```python
from build123d import *

# Parameters (mm, degrees)
SKETCH2_R = 2.5


with BuildPart() as part:
    # Sweep1: sweep along a path in Sketch1
    with BuildLine(Plane(origin=(0, 0, 0), x_dir=(1, 0, 0), z_dir=(0, 1, 0))) as sweep1_path:
        Line((0, 0), (0, 65))
        ThreePointArc((0, 65), (4.393398282, 75.606601718), (15, 80))
        Line((15, 80), (215, 80))
        ThreePointArc((215, 80), (225, 70), (215, 60))
        Line((215, 60), (185, 60))
        ThreePointArc((185, 60), (172.034701688, 62.946330384), (161.616073533, 71.206597355))
    # Sketch2 → Sweep1 (sweep)
    with BuildSketch(Plane.XY):
        Circle(SKETCH2_R)
    sweep(path=sweep1_path.line)


solid = part.part
```
Read the model definition and answer for the solid it produces. Units are mm, in the model's axes. A direction names the side the tool comes from. Round coordinates to 2 decimals unless told otherwise and drop trailing zeros. Write each loop counter-clockwise with the first axis right and the second up, starting at its lowest first coordinate (ties: lowest second). Pieces come first, ordered by that corner, then holes. Notation, with made-up numbers: (35, 74) -> (86, 74) arc R17 ccw to (86, 101) -> close; hole circle Ø8 at (55, 35.25). An arc over 180 degrees is marked (long way). Answer in a Markdown table with one row per item. Add a question column.
1) Given P1, Ø1.5, axis at x = 93, y = -1, coming from the -Z side, flat-ended and moving along its own axis, determine where the tip first touches the part or whether it passes through.
2) Which of the six approach directions +Z, -Z, +X, -X, +Y, -Y give full straight-line access (tool end or side, diameter ignored) to faces 1 (the face through (161.589, 0.035, -71.185)), 2 (the face through (116.4, -0.1, -82.5))?
3) Find section B-B, the plane z = -21.5. Determine the outline of the cut face in (x, y).
4) Find section A-A, the plane y = 0. Determine the outline of the cut face in (x, z).
5) Determine the mould class of faces 3 (the face through (0, 0, 0)), 4 (the face through (-0.54, 2.44, -32.96)), 5 (the face through (199.79, 0.96, -62.31)) for opening direction Z: pulls with the +Z half, pulls with the -Z half, needs draft (parallel to the pull), parting line crosses it, or undercut.
6) Find section C-C, the plane x = 101. Determine the outline of the cut face in (y, z), and give its area (3 significant figures).
7) Consider line 1 (Z direction, x = 19, y = -0.25); line 2 (Y direction, x = 171, z = -62); line 3 (X direction, y = -1.1, z = -21) (3 decimals). Determine where each line is inside the solid, lowest interval first.
Findings below:
| question | item | result |
|---|---|---|
| 1 | P1 | z = -82.49 |
| 2 | face 1 | +Y, -Y |
| 2 | face 2 | none |
| 3 | outline | circle Ø5 at (0, 0) |
| 4 | outline | (-2.5, -65) arc R17.5 ccw to (15, -82.5) -> (215, -82.5) arc R12.5 ccw to (215, -57.5) -> (185, -57.5) arc R32.5 ccw to (159.67, -69.64) -> (163.56, -72.77) arc R27.5 cw to (185, -62.5) -> (215, -62.5) arc R7.5 cw to (215, -77.5) -> (15, -77.5) arc R12.5 cw to (2.5, -65) -> (2.5, 0) -> (-2.5, 0) -> close |
| 5 | face 3 | pulls with the +Z half |
| 5 | face 4 | needs draft |
| 5 | face 5 | undercut |
| 6 | outline | circle Ø5 at (0, -80) |
| 6 | area | 19.6 mm² |
| 7 | line 1 | -82.49 to -77.51 |
| 7 | line 2 | -2.13 to 2.13 |
| 7 | line 3 | -2.245 to 2.245 |
